For this review, use the dimensioned drawing (mm, ordinates from the lowest corner) and the shaded views. A direction names the side the tool comes from. Give positions to 0.01 mm unless a question says otherwise; leave off trailing zeros. Loops run counter-clockwise (first coordinate to the right, second up) from the corner with the lowest first, then second, coordinate; pieces in that order, holes last. Notation, with made-up numbers: (59, -13.75) -> (63, -13.75) arc R23 ccw to (63, 14.25) -> close; hole circle Ø8 at (-8.75, -8). An arc over 180 degrees is marked (long way). Use a Markdown table: item, result. Add a question column.
1. To check wall thickness, follow line 1 (Z direction, x = 33.5, y = 4) (1 decimal); line 2 (X direction, y = 7.25, z = 42); line 3 (X direction, y = 6.75, z = 27). State the ranges of each line that lie inside material, in increasing order.
2. Add section A-A (y = 2.25). State the section outline as (x, z) points (1 decimal).
3. Add section C-C (z = 54.5). State the section outline as (x, y) points.
4. Add section B-B (x = 44). State the section outline as (y, z) points (1 decimal).
5. For the marked faces 1 and 2, list the 3-axis set-ups (+Z, -Z, +X, -X, +Y, -Y) from which the entire face can be reached by the end or side of a thin tool; tool diameter is ignored.
6. For pin 1 Ø1.5 at (y, z) = (4.5, 16) entering from +X; pin 2 Ø12 at (x, z) = (32.5, 37) entering from -Y, all flat-tipped, find the tip position at first contact; note any pin that passes through.
7. Add section D-D (x = 90.5). State the section outline as (y, z) points (1 decimal).
8. Draft analysis for pull direction X (two halves, no side actions). For the marked faces 3, 4 and 5, state which applies: pulls with the +X half, pulls with the -X half, needs draft (parallel to the pull), parting line crosses it, or undercut.
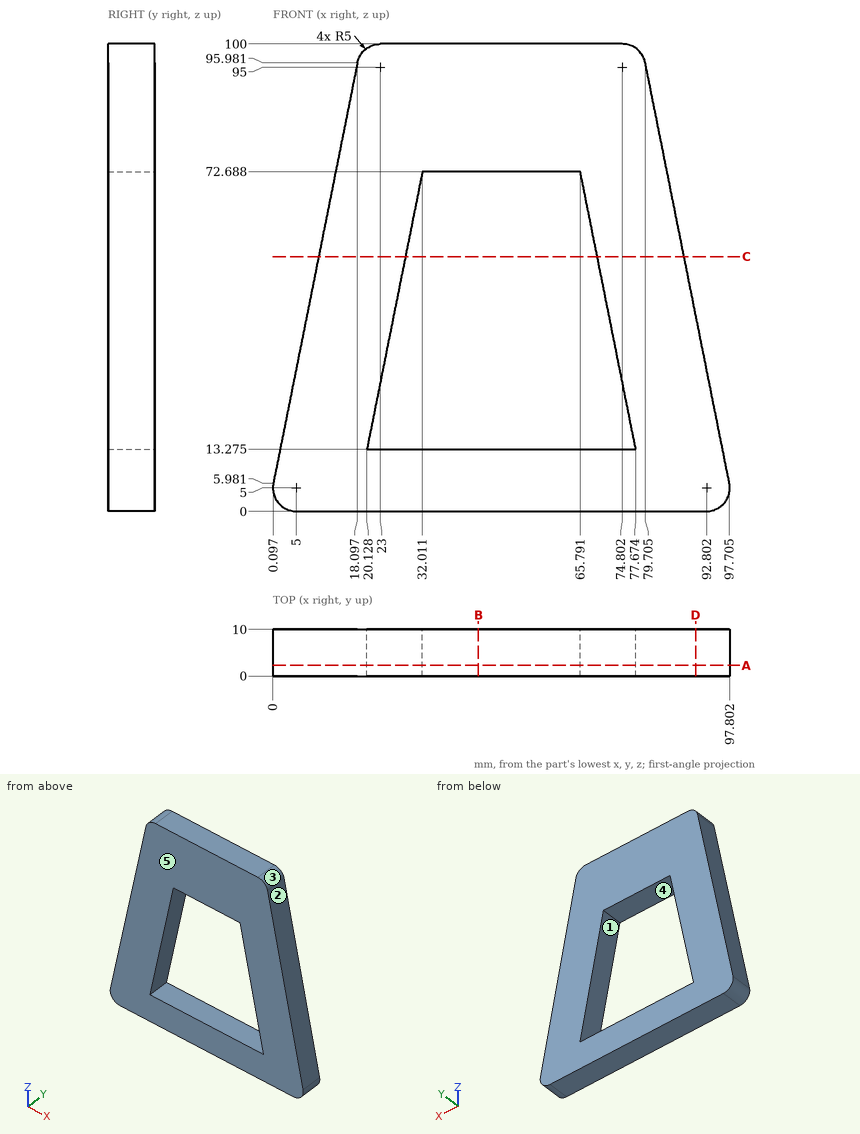
Taken from the geometry:
| question | item | result |
|---|---|---|
| 1 | line 1 | z = 0 to 13.3, 72.7 to 100 |
| 1 | line 2 | x = 7.3 to 25.87, 71.93 to 90.5 |
| 1 | line 3 | x = 4.3 to 22.87, 74.93 to 93.5 |
| 2 | outline | (0.1, 6) arc R5 ccw to (5, 0) -> (92.8, 0) arc R5 ccw to (97.7, 6) -> (79.7, 96) arc R5 ccw to (74.8, 100) -> (23, 100) arc R5 ccw to (18.1, 96) -> close; hole (20.1, 13.3) -> (77.7, 13.3) -> (65.8, 72.7) -> (32, 72.7) -> close |
| 3 | outline | (9.8, 0) -> (28.37, 0) -> (28.37, 10) -> (9.8, 10) -> close; (69.43, 0) -> (88, 0) -> (88, 10) -> (69.43, 10) -> close |
| 4 | outline | (0, 0) -> (10, 0) -> (10, 13.3) -> (0, 13.3) -> close; (0, 72.7) -> (10, 72.7) -> (10, 100) -> (0, 100) -> close |
| 5 | face 1 | +Y, -Y |
| 5 | face 2 | +Z, +X, +Y, -Y |
| 6 | pin 1 | stops at x = 95.85 |
| 6 | pin 2 | passes through |
| 7 | outline | (0, 0) -> (10, 0) -> (10, 42) -> (0, 42) -> close |
| 8 | face 3 | pulls with the +X half |
| 8 | face 4 | undercut |
| 8 | face 5 | needs draft |
